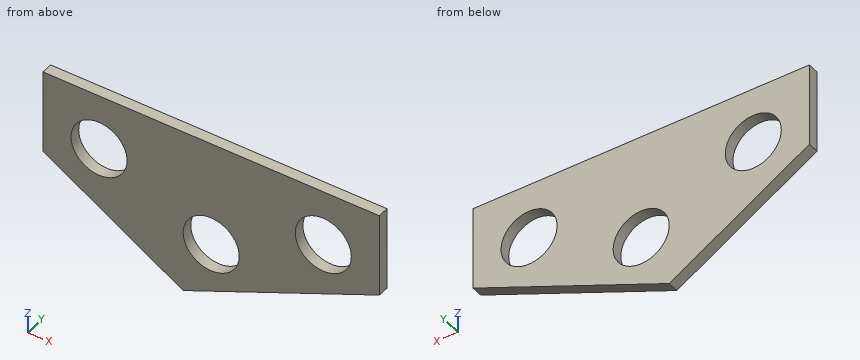
from build123d import *

# Parameters (mm, degrees)
SKETCH1_W           = 60
SKETCH1_H           = 30
BOSS_EXTRUDE1_DEPTH = 2
CUT_EXTRUDE1_DEPTH  = 68.111846942
SKETCH3_R           = 5
CUT_EXTRUDE2_DEPTH  = 68.111846942


with BuildPart() as part:
    # Sketch1 → Boss-Extrude1 (new body)
    with BuildSketch(Plane(origin=(0, 0, 0), x_dir=(1, 0, 0), z_dir=(0, 1, 0))):
        with Locations((30, 15)):
            Rectangle(SKETCH1_W, SKETCH1_H)
    extrude(amount=BOSS_EXTRUDE1_DEPTH)

    # Sketch2 → Cut-Extrude1 (cut, through all)
    with BuildSketch(Plane(origin=(0, 2, 0), x_dir=(1, 0, 0), z_dir=(0, 1, 0))):
        Polygon((60, 15), (60, 30), (25, 30), align=None)
        Polygon((0, 15), (25, 30), (0, 30), align=None)
    extrude(amount=-CUT_EXTRUDE1_DEPTH, mode=Mode.SUBTRACT)

    # Sketch3 → Cut-Extrude2 (cut, through all)
    with BuildSketch(Plane.XZ):
        with Locations(Location((10, -10, 0), (0, 0, 270))):
            Circle(SKETCH3_R)
        with Locations(Location((50, -10, 0), (0, 0, 90))):
            Circle(SKETCH3_R)
        with Locations(Location((30, -19, 0), (0, 0, 270))):
            Circle(SKETCH3_R)
    extrude(amount=-CUT_EXTRUDE2_DEPTH, mode=Mode.SUBTRACT)


solid = part.part
Geometry check sheet. Reference: the model listing, model coordinates, mm. Round coordinates to 2 decimals unless told otherwise and drop trailing zeros. Write each loop counter-clockwise with the first axis right and the second up, starting at its lowest first coordinate (ties: lowest second). Pieces come first, ordered by that corner, then holes.
Item 1: Section check D-D (z = -19). Record the boundary of the cut face in (x, y), plus the area to 3 significant figures.
Determined:
outline: (6.67, 0) - (25, 0) - (25, 2) - (6.67, 2) - close; (35, 0) - (50.67, 0) - (50.67, 2) - (35, 2) - close
area: 68.0 mm2
Item 2: Section check B-B (y = 0.75). Record the boundary of the cut face in (x, z), plus the area to 3 significant figures.
Determined:
outline: (0, -15) - (25, -30) - (60, -15) - (60, 0) - (0, 0) - close; hole circle Ø10 at (10, -10); hole circle Ø10 at (30, -19); hole circle Ø10 at (50, -10)
area: 1,110 mm2
Item 3: Section check C-C (z = -10). Record the boundary of the cut face in (x, y), plus the area to 3 significant figures.
Determined:
outline: (0, 0) - (5, 0) - (5, 2) - (0, 2) - close; (15, 0) - (45, 0) - (45, 2) - (15, 2) - close; (55, 0) - (60, 0) - (60, 2) - (55, 2) - close
area: 80.0 mm2
Item 4: Section check A-A (x = 14). Record the boundary of the cut face in (y, z).
Determined:
outline: (0, -23.4) - (2, -23.4) - (2, -13) - (0, -13) - close; (0, -7) - (2, -7) - (2, 0) - (0, 0) - close
Item 5: Material ranges on line 1 along X through (y, z) = (0.45, -10); line 2 along X through (y, z) = (0.3, -12); line 3 along X through (y, z) = (0.3, -16), recorded low to high.
Determined:
line 1: x = 0 to 5, 15 to 45, 55 to 60
line 2: x = 0 to 5.42, 14.58 to 45.42, 54.58 to 60
line 3: x = 1.67 to 26, 34 to 57.67
Item 6: Go/stop test with flat-tipped pins: pin 1 Ø1 at (x, y) = (53, 1.5) entering from -Z; pin 2 Ø1.5 at (x, z) = (32.5, -18.5) entering from -Y. Record where each tip stops, or that it passes through.
Determined:
pin 1: stops at z = -18.21
pin 2: passes through
